Read the model definition and answer for the solid it produces. Units are mm, in the model's axes. A direction names the side the tool comes from. Give positions to 0.01 mm unless a question says otherwise; leave off trailing zeros. Order: outer loops, then holes, each group sorted by start corner. A loop starts at its lowest first (then second) coordinate and runs counter-clockwise, first axis right, second up. Notation, with made-up numbers: M 57,-26 L 110,-26 A13 ccw 110,-6 Z; hole C 31,58 d2. An arc over 180 degrees is marked long. One line per item, written item: value.
from build123d import *

# Parameters (mm, degrees)
SKETCH1_W                = 30
SKETCH1_H                = 5
BOSS_EXTRUDE2_DEPTH      = 1
BOSS_EXTRUDE3_DEPTH      = 1
BOSS_EXTRUDE3_DEPTH_BACK = 3
SKETCH2_R                = 3
SKETCH2_R_2              = 5
SKETCH3_R                = 1.5
SKETCH3_R_2              = 2.25
CUT_EXTRUDE1_DEPTH       = 41
FILLET1_R                = 0.5
FILLET2_R                = 0.5


with BuildPart() as part:
    # Sketch1 → Boss-Extrude2 (new, symmetric)
    with BuildSketch(Plane(origin=(0, 0, 0), x_dir=(1, 0, 0), z_dir=(0, 1, 0))):
        Rectangle(SKETCH1_W, SKETCH1_H)
    extrude(amount=BOSS_EXTRUDE2_DEPTH, both=True)

    # Sketch2 → Boss-Extrude3 (add, two sides: drawn at the far end of the back side and taken through both)
    with BuildSketch(Plane(origin=(0, 1, 0), x_dir=(1, 0, 0), z_dir=(0, 1, 0)).offset(-BOSS_EXTRUDE3_DEPTH_BACK)):
        with Locations(Location((-15, 0, 0), (0, 0, 270))):
            Circle(SKETCH2_R)
        with Locations(Location((15, 0, 0), (0, 0, 270))):
            Circle(SKETCH2_R_2)
    extrude(amount=BOSS_EXTRUDE3_DEPTH + BOSS_EXTRUDE3_DEPTH_BACK)

    # Sketch3 → Cut-Extrude1 (cut)
    with BuildSketch(Plane(origin=(0, 2, 0), x_dir=(1, 0, 0), z_dir=(0, 1, 0))):
        with Locations(Location((-15, 0, 0), (0, 0, 270))):
            Circle(SKETCH3_R)
        with Locations(Location((15, 0, 0), (0, 0, 270))):
            Circle(SKETCH3_R_2)
    extrude(amount=-CUT_EXTRUDE1_DEPTH, mode=Mode.SUBTRACT)

    # Fillet1
    # the kernel refuses this fillet: 0.5 mm, written as the material it takes off along each edge
    with BuildSketch(Plane(origin=(-14.591687605, 1, 2.5), x_dir=(0, -1, 0), z_dir=(1, 0, 0))) as fillet1_piece_1_section:
        with BuildLine():
            CenterArc((FILLET1_R, FILLET1_R), FILLET1_R, 180, 90)
            Line((0, FILLET1_R), (0, 0))
            Line((0, 0), (FILLET1_R, 0))
        make_face()
    fillet1_piece_1 = extrude(amount=26.511560586, mode=Mode.PRIVATE)
    fillet1_piece_1 = fillet1_piece_1 - Plane(origin=(-15, 0.886280148, 0), x_dir=(0, 0, 1), z_dir=(0, 1, 0)) * Cylinder(3, 56, mode=Mode.PRIVATE)
    fillet1_piece_1 = fillet1_piece_1 - Plane(origin=(15, 0.886280148, 0), x_dir=(0, 0, 1), z_dir=(0, 1, 0)) * Cylinder(5, 56, mode=Mode.PRIVATE)
    add(fillet1_piece_1, mode=Mode.SUBTRACT)
    with BuildSketch(Plane(origin=(11.919872981, 1, -2.5), x_dir=(0, 0, 1), z_dir=(-1, 0, 0))) as fillet1_piece_2_section:
        with BuildLine():
            CenterArc((FILLET1_R, -FILLET1_R), FILLET1_R, 90, 90)
            Line((0, -FILLET1_R), (0, 0))
            Line((0, 0), (FILLET1_R, 0))
        make_face()
    fillet1_piece_2 = extrude(amount=26.511560586, mode=Mode.PRIVATE)
    fillet1_piece_2 = fillet1_piece_2 - Plane(origin=(-15, 0.88627951, 0), x_dir=(0, 0, 1), z_dir=(0, 1, 0)) * Cylinder(3, 56, mode=Mode.PRIVATE)
    fillet1_piece_2 = fillet1_piece_2 - Plane(origin=(15, 0.88627951, 0), x_dir=(0, 0, 1), z_dir=(0, -1, 0)) * Cylinder(5, 56, mode=Mode.PRIVATE)
    add(fillet1_piece_2, mode=Mode.SUBTRACT)

    # Fillet2
    fillet2_edges = [part.edges().sort_by_distance(p)[0] for p in [
        (-1.335907312, -1, 2.5),
        (-1.335907312, -1, -2.5),
    ]]
    fillet(fillet2_edges, radius=FILLET2_R)


solid = part.part
1) Which of the six approach directions +Z, -Z, +X, -X, +Y, -Y give full straight-line access (tool end or side, diameter ignored) to faces 4 (the face through (14, -2, 2.2)), 5 (the face through (-2, 0, 2.5))?
Reported:
face 4: +Z, -Z, +X, -X, -Y
face 5: +Z, +Y, -Y
2) Each of these flat-tipped pins is pushed along its axis until it touches: pin 1 Ø0.5 at (x, y) = (4.5, 0) entering from -Z; pin 2 Ø1.5 at (y, z) = (1.5, -1.5) entering from +X; pin 3 Ø3 at (x, z) = (0, 0.5) entering from -Y. Where does it stop, or does it pass through?
Reported:
pin 1: stops at z = -2.5
pin 2: stops at x = 19.94
pin 3: stops at y = -1
3) Consider probe 1 along X at (y, z) = (0.5, 0); probe 2 along X at (y, z) = (1.2, 0); probe 3 along X at (y, z) = (-1.6, -1). Determine where each line is inside the solid, lowest interval first.
Reported:
probe 1: x = -18 to -16.5, -13.5 to 12.75, 17.25 to 20
probe 2: x = -18 to -16.5, -13.5 to -12, 10 to 12.75, 17.25 to 20
probe 3: x = -17.83 to -16.12, -13.88 to -12.17, 10.1 to 12.98, 17.02 to 19.9
4) Find section D-D, the plane y = 0.05. Write down the section's boundary in (x, z).
Reported:
outline: M -13.34,-2.5 L 10.67,-2.5 A5 ccw long 10.67,2.5 L -13.34,2.5 A3 ccw long Z; hole C -15,0 d3; hole C 15,0 d4.5
5) Determine the mould class of faces 1 (the face through (-14.55, 0.03, 1.43)), 2 (the face through (-2, 0, -2.5)), 3 (the face through (14, 2, 2.2)) for opening direction X: +X half, -X half, draft (parallel to the pull), parting line (faces both ways), or undercut.
Reported:
face 1: undercut
face 2: undercut
face 3: draft
6) Find section A-A, the plane x = -15. Write down the section's boundary in (y, z), plus the area to 3 significant figures.
Reported:
outline: M -2,-3 L 2,-3 L 2,-1.5 L -2,-1.5 Z; M -2,1.5 L 2,1.5 L 2,3 L -2,3 Z
area: 12.0 mm^2
7) Find section B-B, the plane z = 0. Write down the section's boundary in (x, y).
Reported:
outline: M -18,-2 L -16.5,-2 L -16.5,2 L -18,2 Z; M -13.5,-2 L -12,-2 L -12,-1 L 10,-1 L 10,-2 L 12.75,-2 L 12.75,2 L 10,2 L 10,1 L -12,1 L -12,2 L -13.5,2 Z; M 17.25,-2 L 20,-2 L 20,2 L 17.25,2 Z
8) Find section C-C, the plane x = 6.5. Write down the section's boundary in (y, z), plus the area to 3 significant figures.
Reported:
outline: M -1,-2 A0.5 ccw -0.5,-2.5 L 0.5,-2.5 A0.5 ccw 1,-2 L 1,2 A0.5 ccw 0.5,2.5 L -0.5,2.5 A0.5 ccw -1,2 Z
area: 9.79 mm^2
